```python
from build123d import *

# Parameters (mm, degrees)
BOX005_W         = 0.75
BOX005_H         = 10
BOX005_DEPTH     = 0.75
BOX006_W         = 0.75
BOX006_H         = 10
BOX006_DEPTH     = 0.75
BOX007_W         = 0.75
BOX007_H         = 10
BOX007_DEPTH     = 0.75
BOX004_W         = 7
BOX004_H         = 2.5
BOX004_DEPTH     = 4
SKETCH006_R      = 1.5
EXTRUDE003_DEPTH = 2
SKETCH005_R      = 1.5
EXTRUDE002_DEPTH = 1.5
SKETCH007_W      = 4
SKETCH007_H      = 6.5
EXTRUDE004_DEPTH = 8


with BuildPart() as cube001:
    # Box005 → Box005 (new body)
    with BuildSketch(Plane(origin=(2.75, 9, -4), x_dir=(1, 0, 0), z_dir=(0, 0, 1))):
        with Locations((0.375, 5)):
            Rectangle(BOX005_W, BOX005_H)
    extrude(amount=BOX005_DEPTH)


with BuildPart() as cube002:
    # Box006 → Box006 (new body)
    with BuildSketch(Plane(origin=(-0.25, 9, -4), x_dir=(1, 0, 0), z_dir=(0, 0, 1))):
        with Locations((0.375, 5)):
            Rectangle(BOX006_W, BOX006_H)
    extrude(amount=BOX006_DEPTH)


with BuildPart() as cube003:
    # Box007 → Box007 (new body)
    with BuildSketch(Plane(origin=(-3.5, 9, -4), x_dir=(1, 0, 0), z_dir=(0, 0, 1))):
        with Locations((0.375, 5)):
            Rectangle(BOX007_W, BOX007_H)
    extrude(amount=BOX007_DEPTH)


with BuildPart() as fusion005:
    # Box004 → Box004 (new body)
    with BuildSketch(Plane(origin=(-3.5, 9, -4), x_dir=(1, 0, 0), z_dir=(0, 0, 1))):
        with Locations((3.5, 1.25)):
            Rectangle(BOX004_W, BOX004_H)
    extrude(amount=BOX004_DEPTH)

    # Fusion005: union Cube001, Cube002, Cube003
    add(cube001.part)
    add(cube002.part)
    add(cube003.part)


with BuildPart() as extrude003:
    # Sketch006 → Extrude003 (new body)
    with BuildSketch(Plane.XY):
        with BuildLine():
            ThreePointArc((-10, 3.25), (-13.25, 0), (-10, -3.25))
            Line((-10, -3.25), (10, -3.25))
            ThreePointArc((10, -3.25), (13.25, 0), (10, 3.25))
            Line((10, 3.25), (-10, 3.25))
        make_face()
        with Locations((-10, 0)):
            Circle(SKETCH006_R, mode=Mode.SUBTRACT)
        with Locations((10, 0)):
            Circle(SKETCH006_R, mode=Mode.SUBTRACT)
    extrude(amount=EXTRUDE003_DEPTH)


with BuildPart() as extrude003_1:
    # Extrude003 placement: moved
    add(extrude003.part.moved(Location((0, 0, 1.5))))


with BuildPart() as fusion003:
    # Sketch005 → Extrude002 (new body)
    with BuildSketch(Plane.XY):
        with BuildLine():
            Line((-6.25, 11.5), (6.25, 11.5))
            Line((6.25, 11.5), (6.25, 3.5))
            Line((6.25, 3.5), (10, 3.5))
            ThreePointArc((10, -3.5), (13.5, 0), (10, 3.5))
            Line((10, -3.5), (-10, -3.5))
            ThreePointArc((-10, 3.5), (-13.5, 0), (-10, -3.5))
            Line((-10, 3.5), (-6.25, 3.5))
            Line((-6.25, 3.5), (-6.25, 11.5))
        make_face()
        with Locations((-10, 0)):
            Circle(SKETCH005_R, mode=Mode.SUBTRACT)
        with Locations((10, 0)):
            Circle(SKETCH005_R, mode=Mode.SUBTRACT)
    extrude(amount=EXTRUDE002_DEPTH)

    # Fusion003: union Extrude003
    add(extrude003_1.part)


with BuildPart() as extrude004:
    # Sketch007 (on Face15 of Fusion003) → Extrude004 (new body)
    with BuildSketch(Plane.XY.offset(3.5)):
        with Locations((5, 0)):
            Rectangle(SKETCH007_W, SKETCH007_H)
        with Locations((-5, 0)):
            Rectangle(SKETCH007_W, SKETCH007_H)
    extrude(amount=EXTRUDE004_DEPTH)


with BuildPart() as fusion006:
    # Fusion004 base: copy of Fusion003
    add(fusion003.part)

    # Fusion004: union Extrude004
    add(extrude004.part)

    # Fusion006: union Fusion005, Fusion003, Extrude004
    add(fusion005.part)
    add(fusion003.part)
    add(extrude004.part)


solid = fusion006.part
```
Here's how the part is built. I have some questions about the finished solid (model axes, mm). A direction names the side the tool comes from. Give positions to 0.01 mm unless a question says otherwise; leave off trailing zeros. Write each loop counter-clockwise with the first axis right and the second up, starting at its lowest first coordinate (ties: lowest second). Pieces come first, ordered by that corner, then holes. Notation, with made-up numbers: M 71,86.25 L 125,86.25 A25 cw 125,101.25 Z; hole C -26,-28.5 d1. An arc over 180 degrees is marked long. Put each result on its own line as item: value. Start each with the question number.
Item 1: If we section it at A-A, the plane z = 8: Write out the boundary of the cut face in (x, y).
Item 2: I need wall thicknesses on L1, parallel to Y at x = 10, z = 2.35; L2, parallel to X at y = 1.25, z = 6.25; L3, parallel to Y at x = -10, z = 1.4. Which ranges of each line are inside material? Lowest first, please. Write a range as from..to.
Item 3: If we section it at D-D, the plane x = 11: Write out the boundary of the cut face in (y, z).
Item 4: Thinking about a two-plate mould opening in X: for faces 5 (the cylindrical face through (-13.25, 0.07, 2.49)), 6 (the flat face through (-8, 3.5, 1)), 7 (the cylindrical face through (-11.5, 0.07, 1.73)), which applies, +X half, -X half, draft (parallel to the pull), parting line (faces both ways), or undercut?
Item 5: If we section it at B-B, the plane y = 0: Write out the boundary of the cut face in (x, z).
Item 6: On a 3-axis mill with a long thin cutter (end or side, diameter ignored), from which of +Z, -Z, +X, -X, +Y, -Y can I reach the whole of each face in a straight line? I mean faces 1 (the flat face through (7, 0, 7)), 2 (the flat face through (6.25, 8, 1)), 3 (the flat face through (0, -3.25, 3)), 4 (the cylindrical face through (13.25, -0.07, 2.49)). Say none if no direction works.
Item 7: Will these pins go through, and if not, where does the flat tip stop? pin 1 (1.2 mm diameter, centred on x = -7.5, z = 0.5, fed in from +Y); pin 2 (1.5 mm diameter, centred on x = -5.5, y = 6.5, fed in from -Z); pin 3 (2 mm diameter, centred on x = -0.5, y = 3, fed in from +Z); pin 4 (1.9 mm diameter, centred on x = 9.5, y = 0, fed in from +Z).
Item 8: If we section it at C-C, the plane y = 10.5: Write out the boundary of the cut face in (x, z), then the cut area to 4 significant figures.
Values:
1. outline: M -7,-3.25 L -3,-3.25 L -3,3.25 L -7,3.25 Z; M 3,-3.25 L 7,-3.25 L 7,3.25 L 3,3.25 Z
2. L1: -3.25..-1.5, 1.5..3.25
2. L2: -7..-3, 3..7
2. L3: -3.5..-1.5, 1.5..3.5
3. outline: M -3.35,0 L -1.12,0 L -1.12,3.5 L -3.09,3.5 L -3.09,1.5 L -3.35,1.5 Z; M 1.12,0 L 3.35,0 L 3.35,1.5 L 3.09,1.5 L 3.09,3.5 L 1.12,3.5 Z
4. face 5: -X half
4. face 6: draft
4. face 7: undercut
5. outline: M -13.5,0 L -11.5,0 L -11.5,3.5 L -13.25,3.5 L -13.25,1.5 L -13.5,1.5 Z; M -8.5,0 L 8.5,0 L 8.5,3.5 L 7,3.5 L 7,11.5 L 3,11.5 L 3,3.5 L -3,3.5 L -3,11.5 L -7,11.5 L -7,3.5 L -8.5,3.5 Z; M 11.5,0 L 13.5,0 L 13.5,1.5 L 13.25,1.5 L 13.25,3.5 L 11.5,3.5 Z
6. face 1: +Z, +X, +Y, -Y
6. face 2: +Z, -Z, +X, +Y
6. face 3: +Z, +X, -X, -Y
6. face 4: +Z, +X
7. pin 1: y = 3.5
7. pin 2: z = 0
7. pin 3: z = 3.5
7. pin 4: through
8. outline: M -6.25,0 L -3.5,0 L -3.5,-4 L 3.5,-4 L 3.5,0 L 6.25,0 L 6.25,1.5 L -6.25,1.5 Z
8. area: 46.75 mm²
